Part model, mm, in its own coordinate system. Face numbers are marked on the shaded views. A direction names the side the tool comes from. Coordinates: 2 decimals unless noted, no trailing zeros. Loops run counter-clockwise (first coordinate to the right, second up) from the corner with the lowest first, then second, coordinate; pieces in that order, holes last. Notation, with made-up numbers: (7, 55.5) -> (34, 55.5) arc R35 ccw to (34, 88.5) -> close; hole circle Ø6 at (40, 0.25). An arc over 180 degrees is marked (long way). One line per question, with ' | ' between items. Start each with the question number.
1) Probe L1, parallel to Y at x = 0, z = 5.5; L2, parallel to Y at x = -1.5, z = 5.25; L3, parallel to X at y = -6.25, z = 8.25. List the from-to ranges inside material, lowest first. Write a range as from..to.
2) Cut at D-D (z = 2.5). List the corners of the cut face in (x, y), plus the area to 3 significant figures.
3) Cut at B-B (y = 0). List the corners of the cut face in (x, z), plus the area to 3 significant figures.
4) Two-plate mould, pull along Y, no slides. Class the marked faces 3, 4 and 5: released by +Y, released by -Y, zero draft, split by the parting line, or undercut.
5) Drop flat-ended pins along their axis: pin 1 (1 mm diameter, centred on y = 2.5, z = 10.5, fed in from +X); pin 2 (12 mm diameter, centred on x = -5.5, y = 8, fed in from +Z); pin 3 (3 mm diameter, centred on y = -2.5, z = 7, fed in from -X). Give the stop position or say it passes through.
6) Cut at A-A (z = 10.5). List the corners of the cut face in (x, y).
7) 3-axis set-ups, long thin cutter, end or side, ignore diameter. For the marked faces 1 and 2: which of +Z, -Z, +X, -X, +Y, -Y reach the whole face in a straight line?
from build123d import *

# Parameters (mm, degrees)
SKETCH1_R           = 12.5095
SKETCH1_R_2         = 6.9215
BOSS_EXTRUDE1_DEPTH = 12
FILLET1_R           = 1
SKETCH2_R           = 10.7715
SKETCH2_R_2         = 8.8665
CUT_EXTRUDE1_DEPTH  = 9


with BuildPart() as part:
    # Sketch1 → Boss-Extrude1 (new body)
    with BuildSketch(Plane.XY):
        Circle(SKETCH1_R)
        Circle(SKETCH1_R_2, mode=Mode.SUBTRACT)
    extrude(amount=BOSS_EXTRUDE1_DEPTH)

    # Fillet1
    fillet1_edges = [part.edges().sort_by_distance(p)[0] for p in [
        (-12.5095, 0, 0),
        (-6.9215, 0, 0),
    ]]
    fillet(fillet1_edges, radius=FILLET1_R)

    # Sketch2 → Cut-Extrude1 (cut)
    with BuildSketch(Plane.XY.offset(12)):
        Circle(SKETCH2_R)
        Circle(SKETCH2_R_2, mode=Mode.SUBTRACT)
    extrude(amount=-CUT_EXTRUDE1_DEPTH, mode=Mode.SUBTRACT)


solid = part.part
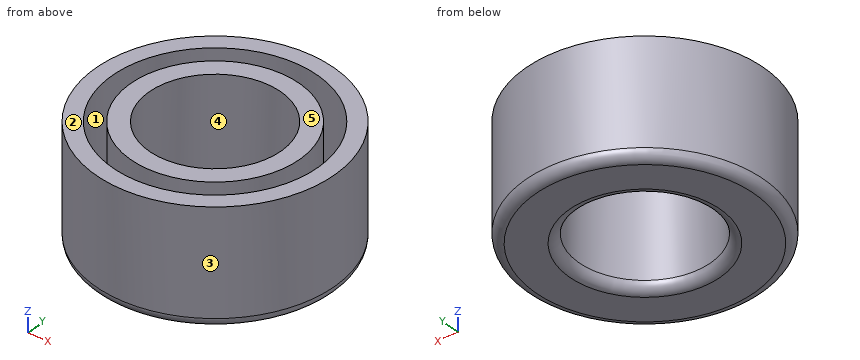
Reported:
1) L1: y = -12.51..-10.77, -8.87..-6.92, 6.92..8.87, 10.77..12.51 | L2: y = -12.42..-10.67, -8.74..-6.76, 6.76..8.74, 10.67..12.42 | L3: x = -10.84..-8.77, -6.29..-2.97, 2.97..6.29, 8.77..10.84
2) outline: circle Ø25.02 at (0, 0); hole circle Ø13.84 at (0, 0) | area: 341 mm²
3) outline: (-12.51, 1) arc R1 ccw to (-11.51, 0) -> (-7.92, 0) arc R1 ccw to (-6.92, 1) -> (-6.92, 12) -> (-8.87, 12) -> (-8.87, 3) -> (-10.77, 3) -> (-10.77, 12) -> (-12.51, 12) -> close; (6.92, 1) arc R1 ccw to (7.92, 0) -> (11.51, 0) arc R1 ccw to (12.51, 1) -> (12.51, 12) -> (10.77, 12) -> (10.77, 3) -> (8.87, 3) -> (8.87, 12) -> (6.92, 12) -> close | area: 99.0 mm²
4) face 3: split by the parting line | face 4: undercut | face 5: zero draft
5) pin 1: stops at x = 12.35 | pin 2: stops at z = 12 | pin 3: stops at x = -12.47
6) outline: circle Ø25.02 at (0, 0); circle Ø17.73 at (0, 0); hole circle Ø21.54 at (0, 0); hole circle Ø13.84 at (0, 0)
7) face 1: +Z | face 2: +Z, +X, -X, +Y, -Y
